from build123d import *

# Parameters (mm, degrees)
F0_W     = 1000
F0_H     = 1000
F1_DEPTH = 25
F2_W     = 100
F2_H     = 300
F3_DEPTH = 200
F4_W     = 200
F4_H     = 700
F4_W_2   = 100
F4_H_2   = 300
F5_DEPTH = 1000
F6_R     = 5


# Not quite as in the source:
# - two fillets or chamfers of one size are made in one step


with BuildPart() as f1:
    # F0 (on Right) → F1 (new body)
    with BuildSketch(Plane.YZ):
        with Locations((334.907528758, 427.1594434977)):
            Rectangle(F0_W, F0_H)
    extrude(amount=F1_DEPTH)

    # F2 (on face) → F3 (join)
    with BuildSketch(Plane.YZ.offset(25)):
        with Locations((334.907528758, 427.1594434977)):
            Rectangle(F2_W, F2_H)
    extrude(amount=F3_DEPTH)

    # F4 (on face) → F5 (join)
    with BuildSketch(Plane.YZ.offset(225)):
        with Locations((334.907528758, 427.1594434977)):
            Rectangle(F4_W, F4_H)
        with Locations((334.907528758, 427.1594434977)):
            Rectangle(F4_W_2, F4_H_2, mode=Mode.SUBTRACT)
        with Locations((334.907528758, 427.1594434977)):
            Rectangle(F4_W_2, F4_H_2)
    extrude(amount=F5_DEPTH)

    # F6
    f6_edges = [f1.edges().sort_by_distance(p)[0] for p in [
        (225, 234.907529, 427.159443),
        (225, 284.907529, 427.159443),
        (725, 234.907529, 777.159443),
        (1225, 234.907529, 427.159443),
        (1225, 334.907529, 777.159443),
        (725, 234.907529, 77.159443),
        (225, 334.907529, 77.159443),
        (1225, 334.907529, 77.159443),
        (225, 334.907529, 777.159443),
        (725, 434.907529, 77.159443),
        (725, 434.907529, 777.159443),
        (225, 434.907529, 427.159443),
        (1225, 434.907529, 427.159443),
    ]]
    fillet(f6_edges, radius=F6_R)


solid = f1.part
Source: CAD feature listing. Evaluate the final solid. Frame: model axes, mm. A direction names the side the tool comes from. Coordinates: 2 decimals unless noted, no trailing zeros. Loops run counter-clockwise (first coordinate to the right, second up) from the corner with the lowest first, then second, coordinate; pieces in that order, holes last. Notation, with made-up numbers: (28, 69.5) - (36, 69.5) arc R28 ccw to (36, 108.5) - close; hole circle Ø8 at (-20.5, 85.5). An arc over 180 degrees is marked (long way). Return JSON: item names as keys, results as strings.
Q1. Section D-D, the plane y = 507. Return loops of the section in (x, z).
Results:
{"outline": "(0, -72.84) - (25, -72.84) - (25, 927.16) - (0, 927.16) - close"}
Q2. Section B-B, the plane z = 385.5. Return loops of the section in (x, y), plus the area to 3 significant figures.
Results:
{"outline": "(0, -165.09) - (25, -165.09) - (25, 284.91) - (220, 284.91) arc R5 cw to (225, 279.91) - (225, 239.91) arc R5 ccw to (230, 234.91) - (1220, 234.91) arc R5 ccw to (1225, 239.91) - (1225, 429.91) arc R5 ccw to (1220, 434.91) - (230, 434.91) arc R5 ccw to (225, 429.91) - (225, 384.91) - (25, 384.91) - (25, 834.91) - (0, 834.91) - close", "area": "245,000 mm2"}
Q3. Section C-C, the plane x = 600. Return loops of the section in (y, z).
Results:
{"outline": "(234.91, 82.16) arc R5 ccw to (239.91, 77.16) - (429.91, 77.16) arc R5 ccw to (434.91, 82.16) - (434.91, 772.16) arc R5 ccw to (429.91, 777.16) - (239.91, 777.16) arc R5 ccw to (234.91, 772.16) - close"}
Q4. Access query for faces 1 (the flat face through (718, 434.908, 422)), 2 (the flat face through (124, 332, 577.159)), 3 (the flat face through (718, 234.908, 422)). Directions: +Z, -Z, +X, -X, +Y, -Y. A direction counts if a zero-diameter tool reaches every point of the face in a straight line with its end or side. Return the directions, or none.
Results:
{"face 1": "+Z, -Z, +X, +Y", "face 2": "+Z, +Y, -Y", "face 3": "+Z, -Z, +X, -Y"}
Q5. Material intervals for line 1 along X through (y, z) = (591.5, 870.5); line 2 along Z through (x, y) = (104, 344.5); line 3 along Z through (x, y) = (998, 271.5), sorted ascending.
Results:
{"line 1": "0 to 25", "line 2": "277.16 to 577.16", "line 3": "77.16 to 777.16"}
Q6. Section A-A, the plane z = 117. Return loops of the section in (x, y).
Results:
{"outline": "(0, -165.09) - (25, -165.09) - (25, 834.91) - (0, 834.91) - close; (225, 239.91) arc R5 ccw to (230, 234.91) - (1220, 234.91) arc R5 ccw to (1225, 239.91) - (1225, 429.91) arc R5 ccw to (1220, 434.91) - (230, 434.91) arc R5 ccw to (225, 429.91) - close"}
Q7. Contact query for flat-ended pins moving along their axis: P1, Ø8, axis at y = 459.5, z = 465.5, coming from the +X side; P2, Ø3, axis at x = 1059.5, z = 687, coming from the -Y side; P3, Ø2, axis at y = 504.5, z = 581, coming from the -X side; P4, Ø10, axis at x = 807.5, z = 748, coming from the +Y side. Output: stop coordinate, or through.
Results:
{"P1": "x = 25", "P2": "y = 234.91", "P3": "x = 0", "P4": "y = 434.91"}
